Autodesk Inventor part; units mm, degrees
ref_plane "YZ Plane" through (0, 0, 0) normal (1, 0, 0) x (0, 1, 0)
ref_plane "XZ Plane" through (0, 0, 0) normal (0, 1, 0) x (-1, 0, 0)
ref_plane "XY Plane" through (0, 0, 0) normal (0, 0, 1) x (1, 0, 0)
sketch "Sketch1" plane through (0, 0, 0) normal (0, 1, 0) x (-1, 0, 0)
  line L0 (4.9, 4.9) -> (-4.9, 4.9)
  line L1 (-4.9, 4.9) -> (-4.9, -4.9)
  line L2 (-4.9, -4.9) -> (4.9, -4.9)
  line L3 (4.9, -4.9) -> (4.9, 4.9)
  line L4 (4.9, 4.9) -> (-4.9, -4.9) construction
  line L5 (-4.9, 4.9) -> (4.9, -4.9) construction
  point P0 (0, 0)
  dimension "d0" = 9.8
  dimension "d1" = 9.8
extrude "Extrusion1" add sketch "Sketch1" against normal blind 3
sketch "Sketch2" plane through (0, -3, 0) normal (0, -1, 0) x (1, 0, 0)
  circle A0 centre (0, 0) radius 10
  dimension "d4" = 20
extrude "Extrusion2" add sketch "Sketch2" along normal blind 30
sketch "Sketch3" plane through (0, -33, 0) normal (0, -1, 0) x (1, 0, 0)
  arc A0 (56.6685, -50.6545) -> (56.6685, -62.6825) centre (56.6685, -56.6685) ccw
  line L0 (56.6685, -56.6685) -> (0, -56.6685)
  line L1 (0, -56.6685) -> (0, 0)
  circle A1 centre (0, 0) radius 10
  circle A2 centre (0, 0) radius 10
  line L2 (0, -56.6685) -> (-5, -56.6685)
  line L3 (-5, -56.6685) -> (-9.9607, -0.8858)
  line L4 (56.6685, 5) -> (0.8858, 9.9607)
  line L5 (0, -56.6685) -> (5, -56.6685)
  line L6 (56.6685, -5) -> (0.8858, -9.9607)
  line L7 (5, -56.6685) -> (9.9607, -0.8858)
  line L8 (56.6685, 5) -> (112.4513, 9.9607)
  line L9 (56.6685, -5) -> (112.4513, -9.9607)
  line L10 (-5, -56.6685) -> (-9.9607, -112.4513)
  line L11 (5, -56.6685) -> (9.9607, -112.4513)
  line L12 (56.6685, 5) -> (56.6685, -5)
  line L13 (56.6685, 0) -> (56.6685, 1.5)
  line L14 (56.6685, 1.5) -> (59.1685, 1.5)
  line L15 (59.1685, 1.5) -> (59.1685, 2.5)
  line L16 (56.6685, 0) -> (56.6685, -1.5)
  line L17 (56.6685, -1.5) -> (59.1685, -1.5)
  line L18 (59.1685, -1.5) -> (59.1685, -2.5)
  line L19 (59.1685, -2.5) -> (61.6685, -2.5)
  line L20 (61.6685, -2.5) -> (61.6685, 2.5)
  line L21 (61.6685, 2.5) -> (59.1685, 2.5)
  line L22 (-1.5, -56.6685) -> (-1.5, -54.1685)
  line L23 (-1.5, -54.1685) -> (-2.5, -54.1685)
  line L24 (1.5, -56.6685) -> (1.5, -54.1685)
  line L25 (1.5, -54.1685) -> (2.5, -54.1685)
  line L26 (2.5, -54.1685) -> (2.5, -51.6685)
  line L27 (2.5, -51.6685) -> (-2.5, -51.6685)
  line L28 (-2.5, -51.6685) -> (-2.5, -54.1685)
  line L29 (-1.5, -56.6685) -> (1.5, -56.6685)
  line L30 (1.5, -56.6685) -> (1.65, -56.6685)
  line L31 (1.65, -56.6685) -> (1.65, -56.5185)
  line L32 (1.65, -56.5185) -> (1.5, -56.5185)
  line L33 (1.5, -56.5185) -> (1.5, -56.6685)
  line L34 (1.5, -54.1685) -> (1.65, -54.1685)
  line L35 (1.65, -54.1685) -> (1.65, -54.3185)
  line L36 (1.65, -54.3185) -> (1.5, -54.3185)
  line L37 (1.5, -54.3185) -> (1.5, -54.1685)
  line L38 (2.5, -54.1685) -> (2.65, -54.1685)
  line L39 (2.65, -54.1685) -> (2.65, -54.3185)
  line L40 (2.65, -54.3185) -> (2.5, -54.3185)
  line L41 (2.5, -54.3185) -> (2.5, -54.1685)
  line L42 (2.5, -51.6685) -> (2.65, -51.6685)
  line L43 (2.65, -51.6685) -> (2.65, -51.5185)
  line L44 (2.65, -51.5185) -> (2.5, -51.5185)
  line L45 (2.5, -51.5185) -> (2.5, -51.6685)
  line L46 (-2.5, -51.6685) -> (-2.65, -51.6685)
  line L47 (-2.65, -51.6685) -> (-2.65, -51.5185)
  line L48 (-2.65, -51.5185) -> (-2.5, -51.5185)
  line L49 (-2.5, -51.5185) -> (-2.5, -51.6685)
  line L50 (-2.5, -54.1685) -> (-2.65, -54.1685)
  line L51 (-2.65, -54.1685) -> (-2.65, -54.3185)
  line L52 (-2.65, -54.3185) -> (-2.5, -54.3185)
  line L53 (-2.5, -54.3185) -> (-2.5, -54.1685)
  line L54 (-1.5, -54.1685) -> (-1.65, -54.1685)
  line L55 (-1.65, -54.1685) -> (-1.65, -54.3185)
  line L56 (-1.65, -54.3185) -> (-1.5, -54.3185)
  line L57 (-1.5, -54.3185) -> (-1.5, -54.1685)
  line L58 (-1.5, -56.6685) -> (-1.65, -56.6685)
  line L59 (-1.65, -56.6685) -> (-1.65, -56.5185)
  line L60 (-1.65, -56.5185) -> (-1.5, -56.5185)
  line L61 (-1.5, -56.5185) -> (-1.5, -56.6685)
  line L62 (2.65, -51.6685) -> (2.65, -54.1685)
  line L63 (2.5, -51.5185) -> (-2.5, -51.5185)
  line L64 (-2.65, -51.6685) -> (-2.65, -54.1685)
  line L65 (-1.65, -54.3185) -> (-2.5, -54.3185)
  line L66 (-1.65, -54.3185) -> (-1.65, -56.5185)
  line L67 (1.65, -54.3185) -> (2.5, -54.3185)
  line L68 (1.65, -54.3185) -> (1.65, -56.5185)
  point P0 (0.8858, 9.9607)
  point P1 (0.8858, -9.9607)
  point P2 (0, -56.6685)
  point P3 (9.2196, -9.2196)
  point P4 (-9.9607, -0.8858)
  dimension "d8" = 5
  dimension "d23" = 1.5
  dimension "d24" = 2.5
  dimension "d25" = 1
  dimension "d26" = 1.5
  dimension "d27" = 2.5
  dimension "d28" = 1
  dimension "d29" = 2.5
  dimension "d32" = 2.5
  dimension "d33" = 1
  dimension "d34" = 2.5
  dimension "d35" = 1
  dimension "d36" = 2.5
  dimension "d37" = 0.15
  dimension "d38" = 0.15
  dimension "d39" = 0.15
  dimension "d40" = 0.15
  dimension "d41" = 0.15
  dimension "d42" = 0.15
  dimension "d43" = 0.15
  dimension "d44" = 0.15
  dimension "d45" = 0.15
  dimension "d46" = 0.15
  dimension "d47" = 0.15
  dimension "d48" = 0.15
  dimension "d49" = 0.15
  dimension "d50" = 0.15
  dimension "d51" = 0.15
  dimension "d52" = 0.15
extrude "Extrusion3" add sketch "Sketch3" along normal blind 10 contours L0 L31 L68 L67 L40 L39 L62 L43 L44 L63 L1 A1 L6 L7 | L7 A1 L4 L12 L6 | L6 A1 L7 | A1 | L12 L14 L15 L21 L20 L19 L18 L17 | L1 L63 L48 L47 L64 L51 L52 L65 L66 L59 L2 L3 A1
properties part number "Leg_v1"
Can you work these out from the model? Positions are in its coordinate system, mm. A direction names the side the tool comes from. Round coordinates to 2 decimals unless told otherwise and drop trailing zeros. Loops run counter-clockwise (first coordinate to the right, second up) from the corner with the lowest first, then second, coordinate; pieces in that order, holes last. Notation, with made-up numbers: M -10.75,-6 L 18.25,-6 A30 ccw 18.25,24 Z; hole C 85,-10 d1. An arc over 180 degrees is marked long. Write item = value, one per line. Start each with the question number.
(1) Which directions (+Z, -Z, +X, -X, +Y, -Y) give clear straight access to the entire face, cutting with the end or side of a thin tool? Please do faces 1 (the face through (0, -38, -51.518)), 2 (the face through (1.65, -38, -56)), 3 (the face through (0, -1, 4.9)), 4 (the face through (60, -38, 2.5)).
(2) I'm going to push flat-ended pins straight in: P1, Ø8, axis at x = 6.5, y = -25.5, coming from the -Z side; P2, Ø2, axis at x = 57.5, y = -36, coming from the -Z side (3 decimals); P3, Ø20, axis at x = 42, z = -10.5, coming from the +Y side; P4, Ø10, axis at x = -2, z = 0.5, coming from the +Y side. Where does each tip first touch, or does it pass through?
(3) Suppose I cut it at D-D on x = 14.5. Write out the boundary of the cut face in (y, z).
(4) Suppose I cut it at A-A on z = 0. Write out the boundary of the cut face in (x, y).
(5) If we mould it in two halves opening along Z, with no side actions, what happens to faces 5 (the face through (-2.65, -38, -53)), 6 (the face through (0, -1, -4.9)), 7 (the face through (15, -43, -8))? For each: released by +Z, released by -Z, zero draft, split by the parting line, or undercut.
(6) Suppose I cut it at B-B on y = -40. Write out the boundary of the cut face in (x, z).
(7) I need wall thicknesses on line 1 along Y through (x, z) = (23.5, -0.5); line 2 along Z through (x, y) = (-1, -19); line 3 along X through (y, z) = (-19, -2). Which ranges of each line are inside material? Lowest first, please.
(8) Suppose I cut it at C-C on x = 0. Write out the boundary of the cut face in (y, z), plus the area to 3 significant figures.
Answer block:
q1.face_1 = +Y, -Y
q1.face_2 = -Z, +Y, -Y
q1.face_3 = +Z, +X, -X, +Y
q1.face_4 = +Z, +X, +Y, -Y
q2.P1 = -9.68
q2.P2 = -5.015
q2.P3 = -33
q2.P4 = 0
q3.outline = M -43,-8.75 L -33,-8.75 L -33,8.75 L -43,8.75 Z
q4.outline = M -10,-43 L 61.67,-43 L 61.67,-33 L 10,-33 L 10,-3 L 4.9,-3 L 4.9,0 L -4.9,0 L -4.9,-3 L -10,-3 Z
q5.face_5 = undercut
q5.face_6 = released by -Z
q5.face_7 = zero draft
q6.outline = M -9.96,-0.89 L -5,-56.67 L -1.65,-56.67 L -1.65,-54.32 L -2.65,-54.32 L -2.65,-51.52 L 2.65,-51.52 L 2.65,-54.32 L 1.65,-54.32 L 1.65,-56.67 L 5,-56.67 L 9.22,-9.22 L 56.67,-5 L 56.67,-1.5 L 59.17,-1.5 L 59.17,-2.5 L 61.67,-2.5 L 61.67,2.5 L 59.17,2.5 L 59.17,1.5 L 56.67,1.5 L 56.67,5 L 0.89,9.96 A10 ccw Z
q7.line_1 = -43 to -33
q7.line_2 = -9.95 to 9.95
q7.line_3 = -9.8 to 9.8
q8.outline = M -43,-51.52 L -33,-51.52 L -33,-10 L -3,-10 L -3,-4.9 L 0,-4.9 L 0,4.9 L -3,4.9 L -3,10 L -43,10 Z
q8.area = 1,240 mm²
